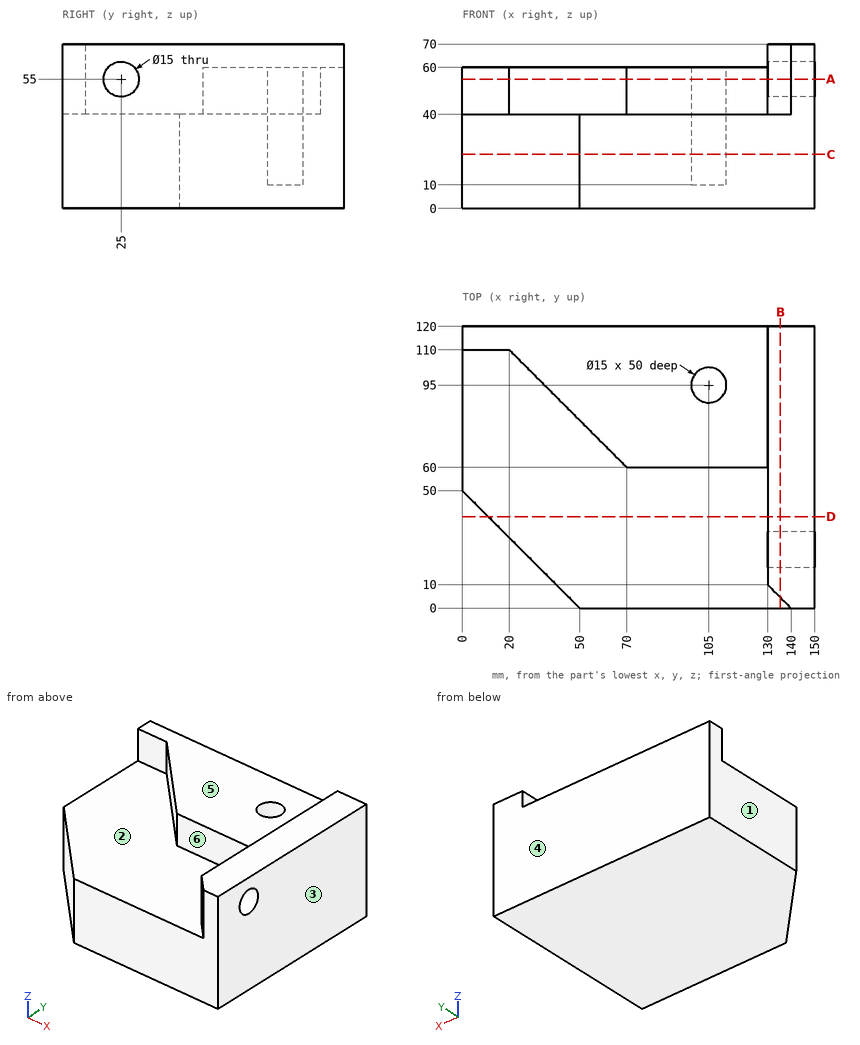
Print and shaded views of the part. All mm, measured from the part's lowest x, y and z. A direction names the side the tool comes from. Give positions to 0.01 mm unless a question says otherwise; leave off trailing zeros. Write each loop counter-clockwise with the first axis right and the second up, starting at its lowest first coordinate (ties: lowest second). Pieces come first, ordered by that corner, then holes. Notation, with made-up numbers: M -16,-27 L 23,-27 A25 cw 23,-12 Z; hole C 79,-24 d7. An arc over 180 degrees is marked long. Use a Markdown table: item, result.
1) Cut at B-B (x = 135.5). List the corners of the cut face in (y, z).
Responses:
| item | result |
|---|---|
| outline | M 0,0 L 120,0 L 120,70 L 4.5,70 L 4.5,40 L 0,40 Z; hole C 25,55 d15 |
2) Drill centre lines: line 1 (Z direction, x = 141.5, y = 25); line 2 (Y direction, x = 105, z = 30); line 3 (X direction, y = 95, z = 32). Where is each one in solid material? Low to high. Write a range as from..to.
Responses:
| item | result |
|---|---|
| line 1 | z = 0..47.5, 62.5..70 |
| line 2 | y = 0..87.5, 102.5..120 |
| line 3 | x = 0..97.5, 112.5..150 |
3) Cut at D-D (y = 39). List the corners of the cut face in (x, z).
Responses:
| item | result |
|---|---|
| outline | M 11,0 L 150,0 L 150,70 L 130,70 L 130,40 L 11,40 Z |
4) Cut at C-C (z = 23). List the corners of the cut face in (x, y), and give its area (3 significant figures).
Responses:
| item | result |
|---|---|
| outline | M 0,50 L 50,0 L 150,0 L 150,120 L 0,120 Z; hole C 105,95 d15 |
| area | 16,600 mm2 |
5) Cut at A-A (z = 55). List the corners of the cut face in (x, y).
Responses:
| item | result |
|---|---|
| outline | M 0,110 L 20,110 L 70,60 L 130,60 L 130,32.5 L 150,32.5 L 150,120 L 0,120 Z; M 130,10 L 140,0 L 150,0 L 150,17.5 L 130,17.5 Z; hole C 105,95 d15 |
6) Pin check, flat tips, straight feed: pin 1 (13.5 mm diameter, centred on x = 105, y = 95, fed in from +Z); pin 2 (9 mm diameter, centred on y = 40, z = 49.5, fed in from -X); pin 3 (12 mm diameter, centred on x = 104.5, y = 98.5, fed in from +Z). Stop position of each tip, or through.
Responses:
| item | result |
|---|---|
| pin 1 | stops at z = 10 |
| pin 2 | stops at x = 130 |
| pin 3 | stops at z = 60 |
7) Pull direction X, two halves, no side cores. Call the marked faces 1, 2 and 3: +X half, -X half, draft (parallel to the pull), parting line (faces both ways), or undercut.
Responses:
| item | result |
|---|---|
| face 1 | -X half |
| face 2 | draft |
| face 3 | +X half |
8) Tool access for the marked faces 4, 5 and 6: list every direction of +Z, -Z, +X, -X, +Y, -Y with a clear straight run to the whole face (end or side of a thin tool).
Responses:
| item | result |
|---|---|
| face 4 | +Z, -Z, +X, -X, +Y |
| face 5 | +Z, -X, +Y, -Y |
| face 6 | +Z, -X, -Y |
